Here's the drawing with two shaded views (mm, measured from the low corner). I have some questions. Coordinates: 2 decimals unless noted, no trailing zeros. Order: outer loops, then holes, each group sorted by start corner. A loop starts at its lowest first (then second) coordinate and runs counter-clockwise, first axis right, second up. Notation, with made-up numbers: (50.5, 12) -> (82.5, 12) arc R15 cw to (82.5, 29) -> close; hole circle Ø6 at (-21, -8.5). An arc over 180 degrees is marked (long way). Answer as a JSON object with one key per item and string values. Group by question number.
(1) I want a section at C-C, the plane z = 131. List the corners of the cut face in (x, y) for me, plus the area to 3 significant figures.
(2) For pin 1 (5 mm diameter, centred on y = 26.5, z = 64, fed in from +X); pin 2 (1.5 mm diameter, centred on y = 31.5, z = 82.5, fed in from -X); pin 3 (10 mm diameter, centred on y = 7, z = 153, fed in from -X) (1 decimal), each with a flat end and sliding along its axis, tell me the tip position at first contact or that it passes through.
(3) I want a section at B-B, the plane y = 4. List the corners of the cut face in (x, z) for me.
(4) I need wall thicknesses on line 1 (X direction, y = 12.5, z = 90.5); line 2 (X direction, y = 35, z = 100) (1 decimal); line 3 (Y direction, x = 221.5, z = 123). Which ranges of each line are inside material? Lowest first, please.
(5) I want a section at D-D, the plane x = 264.5. List the corners of the cut face in (y, z) for me, plus the area to 3 significant figures.
(6) I want a section at A-A, the plane x = 101.5. List the corners of the cut face in (y, z) for me, plus the area to 3 significant figures.
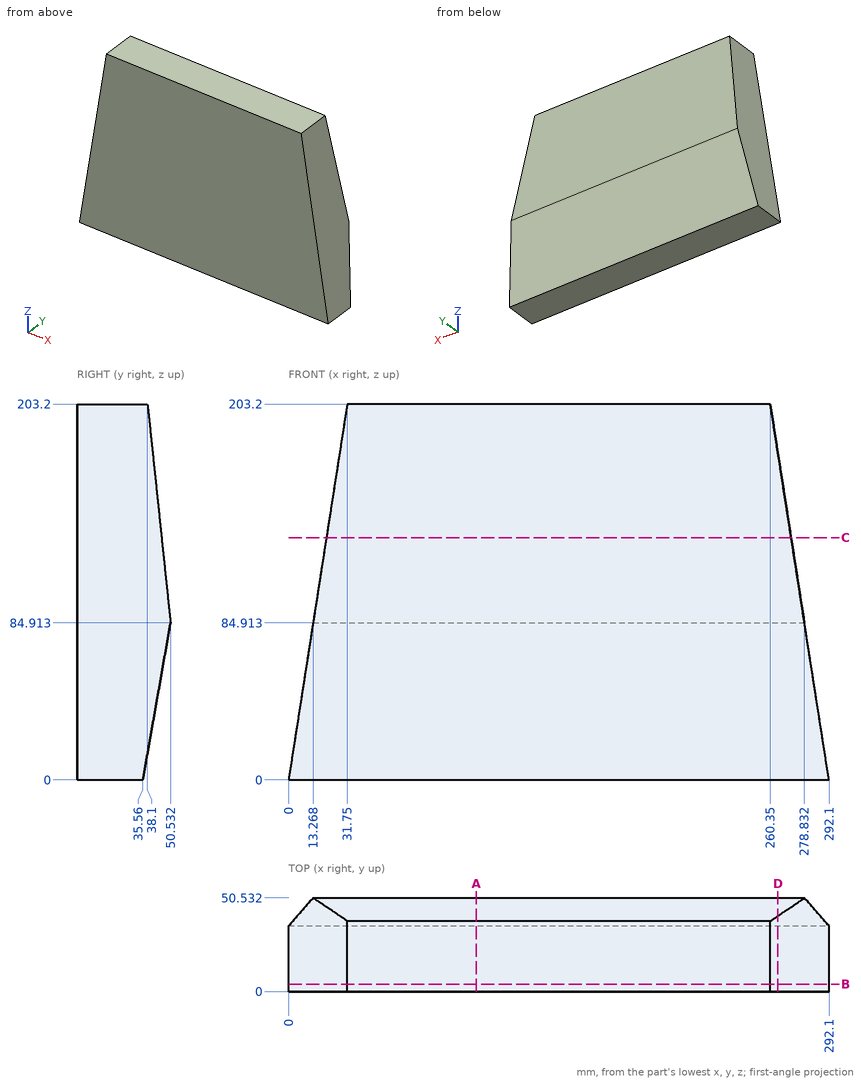
Computed values:
{
 "1": {"outline": "(20.47, 0) -> (271.63, 0) -> (271.63, 45.69) -> (20.47, 45.69) -> close", "area": "11,500 mm2"},
 "2": {"pin 1": "stops at x = 282.49", "pin 2": "stops at x = 12.77", "pin 3": "stops at x = 23.1"},
 "3": {"outline": "(0, 0) -> (292.1, 0) -> (260.35, 203.2) -> (31.75, 203.2) -> close"},
 "4": {"line 1": "x = 14.14 to 277.96", "line 2": "x = 15.6 to 276.5", "line 3": "y = 0 to 46.53"},
 "5": {"outline": "(0, 0) -> (35.56, 0) -> (50.53, 84.91) -> (40.89, 176.64) -> (0, 176.64) -> close", "area": "7,850 mm2"},
 "6": {"outline": "(0, 0) -> (35.56, 0) -> (50.53, 84.91) -> (38.1, 203.2) -> (0, 203.2) -> close", "area": "8,900 mm2"}
}
